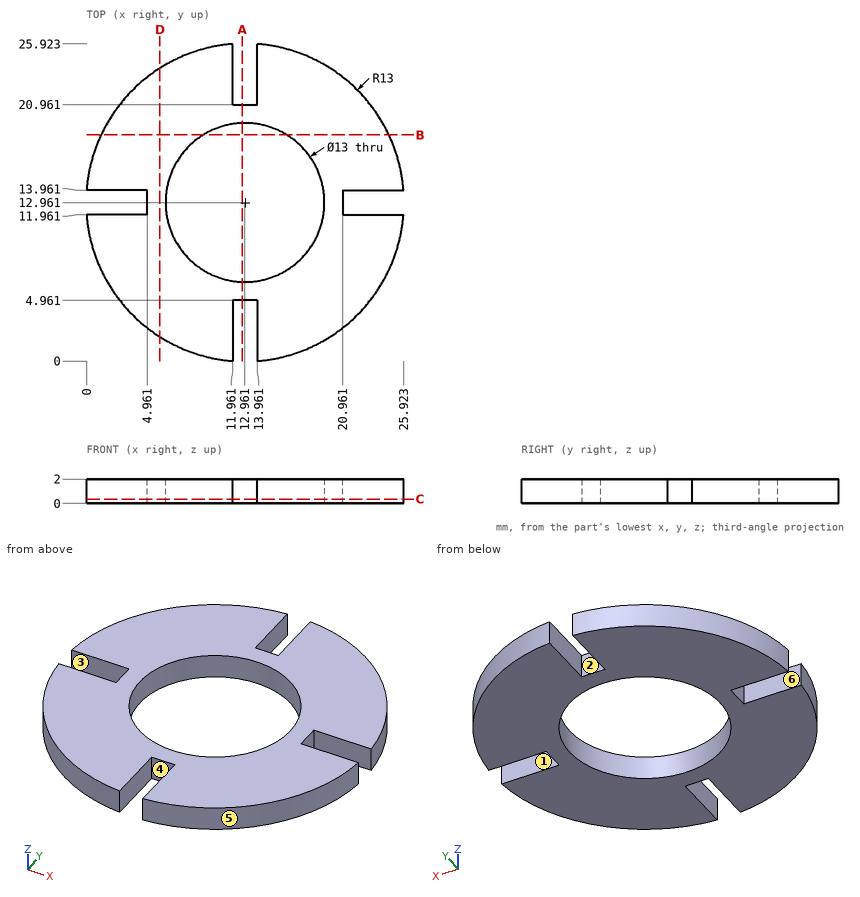
Check sheet for the drawn part. Datum: minimum x, y, z corner. Units: mm. A direction names the side the tool comes from. Round coordinates to 2 decimals unless told otherwise and drop trailing zeros. Order: outer loops, then holes, each group sorted by start corner. A loop starts at its lowest first (then second) coordinate and runs counter-clockwise, first axis right, second up.
(1) Cross-section at D-D, the plane x = 6. Enter the section's corners in (y, z).
(2) Draft check along X on the marked faces 4, 5 and 6. Enter one of: pulls with the +X half, pulls with the -X half, needs draft (parallel to the pull), parting line crosses it, or undercut.
(3) Go/stop test with flat-tipped pins: P1, Ø0.6, axis at x = 22.5, z = 1, coming from the -Y side (1 decimal); P2, Ø0.6, axis at y = 3, z = 1.5, coming from the +X side; P3, Ø1, axis at y = 23.5, z = 1.5, coming from the -X side. Record where each tip stops, or that it passes through.
(4) Access from +Z, -Z, +X, -X, +Y, -Y to the whole of each face (thin tool, end or side, straight path). Record for the marked faces 1, 2 and 3.
(5) Cross-section at C-C, the plane z = 0.35. Enter the section's corners in (x, y).
(6) Scan lines: probe 1 along X at (y, z) = (11.25, 1.2) (1 decimal); probe 2 along Y at (x, z) = (21.5, 1.2) (1 decimal); probe 3 along Y at (x, z) = (1.75, 1.3) (1 decimal). Record each from-to range of solid material in increasing order.
(7) Cross-section at B-B, the plane y = 18.5. Enter the section's corners in (x, z).
(8) Cross-section at A-A, the plane x = 12.75. Enter the section's corners in (y, z) (1 decimal).
Check sheet entries:
1. outline: (1.98, 0) - (23.94, 0) - (23.94, 2) - (1.98, 2) - close
2. face 4: undercut
2. face 5: pulls with the +X half
2. face 6: needs draft
3. P1: stops at y = 3.8
3. P2: stops at x = 21.66
3. P3: stops at x = 4.7
4. face 1: +Z, -Z, +X
4. face 2: +Z, -Z, +Y
4. face 3: +Z, -Z, -X
5. outline: (0, 11.96) arc R13 ccw to (11.96, 0) - (11.96, 4.96) - (13.96, 4.96) - (13.96, 0) arc R13 ccw to (25.92, 11.96) - (20.96, 11.96) - (20.96, 13.96) - (25.92, 13.96) arc R13 ccw to (13.96, 25.92) - (13.96, 20.96) - (11.96, 20.96) - (11.96, 25.92) arc R13 ccw to (0, 13.96) - (4.96, 13.96) - (4.96, 11.96) - close; hole circle Ø13 at (12.96, 12.96)
6. probe 1: x = 0.1 to 6.7, 19.2 to 25.8
6. probe 2: y = 3.2 to 12, 14 to 22.8
6. probe 3: y = 6.4 to 12, 14 to 19.5
7. outline: (1.2, 0) - (9.56, 0) - (9.56, 2) - (1.2, 2) - close; (16.36, 0) - (24.72, 0) - (24.72, 2) - (16.36, 2) - close
8. outline: (5, 0) - (6.5, 0) - (6.5, 2) - (5, 2) - close; (19.5, 0) - (21, 0) - (21, 2) - (19.5, 2) - close
